from build123d import *

# Parameters (mm, degrees)
SKETCH_1_W          = 160
SKETCH_1_H          = 10
EXTRUDE_1_DEPTH     = 2
FILLET_1_R          = 5
CUT_EXTRUDE_1_DEPTH = 10


with BuildPart() as part:
    # 스케치1 → 보스-돌출1 (new body)
    with BuildSketch(Plane(origin=(0, 0, 0), x_dir=(1, 0, 0), z_dir=(0, 1, 0))):
        with Locations((80, 5)):
            Rectangle(SKETCH_1_W, SKETCH_1_H)
    extrude(amount=EXTRUDE_1_DEPTH)

    # 필렛1
    fillet_1_edges = [part.edges().sort_by_distance(p)[0] for p in [
        (0, 1, 0),
        (0, 1, -10),
        (160, 1, -10),
        (160, 1, 0),
    ]]
    fillet(fillet_1_edges, radius=FILLET_1_R - 0.0001)  # a hair under: the kernel refuses the full size

    # 스케치2 → 컷-돌출1 (cut)
    with BuildSketch(Plane(origin=(0, 2, 0), x_dir=(1, 0, 0), z_dir=(0, 1, 0))):
        with BuildLine():
            Line((5, 7.45), (35, 7.45))
            ThreePointArc((35, 7.45), (37.45, 5), (35, 2.55))
            Line((35, 2.55), (5, 2.55))
            ThreePointArc((5, 2.55), (2.55, 5), (5, 7.45))
        make_face()
        with BuildLine():
            Line((45, 7.45), (75, 7.45))
            ThreePointArc((75, 7.45), (77.45, 5), (75, 2.55))
            Line((75, 2.55), (45, 2.55))
            ThreePointArc((45, 2.55), (42.55, 5), (45, 7.45))
        make_face()
        with BuildLine():
            Line((85, 7.45), (115, 7.45))
            ThreePointArc((115, 7.45), (117.45, 5), (115, 2.55))
            Line((115, 2.55), (85, 2.55))
            ThreePointArc((85, 2.55), (82.55, 5), (85, 7.45))
        make_face()
        with BuildLine():
            Line((125, 7.45), (155, 7.45))
            ThreePointArc((155, 7.45), (157.45, 5), (155, 2.55))
            Line((155, 2.55), (125, 2.55))
            ThreePointArc((125, 2.55), (122.55, 5), (125, 7.45))
        make_face()
    extrude(amount=-CUT_EXTRUDE_1_DEPTH, mode=Mode.SUBTRACT)


solid = part.part
Here's how the part is built. I have some questions about the finished solid (model axes, mm). A direction names the side the tool comes from. Coordinates: 2 decimals unless noted, no trailing zeros. Order: outer loops, then holes, each group sorted by start corner. A loop starts at its lowest first (then second) coordinate and runs counter-clockwise, first axis right, second up. Notation, with made-up numbers: M -15.5,-1.75 L -3.5,-1.75 A10 ccw -3.5,17.25 Z; hole C 45.25,-24 d9. An arc over 180 degrees is marked long. Answer as CSV lines item,"result". Start each with the question number.
1. I need wall thicknesses on line 1 (Z direction, x = 144.5, y = 1.2); line 2 (X direction, y = 1.2, z = -5.5). Which ranges of each line are inside material? Lowest first, please. Write a range as [from, to].
2. I want a section at A-A, the plane x = 62.5. Write out the boundary of the cut face in (y, z), and give its area (3 significant figures).
3. We'd pull the mould along X, two halves only. Please class faces 3 (the cylindrical face through (159, 1, -8)), 4 (the cylindrical face through (1, 1, -8)), 5 (the cylindrical face through (122.55, 1.01, -4.95)): released by +X, released by -X, zero draft, split by the parting line, or undercut.
4. On a 3-axis mill with a long thin cutter (end or side, diameter ignored), from which of +Z, -Z, +X, -X, +Y, -Y can I reach the whole of each face in a straight line? I mean faces 1 (the flat face through (79, 2, -5)), 2 (the cylindrical face through (77.45, 1.01, -5.05)). Say none if no direction works.
5. I want a section at B-B, the plane y = 0.6. Count the separate pieces of the cut face and the enclosed holes in it, and give its area (3 significant figures).
Recorded:
1,line 1,"z = [-10, -7.45], [-2.55, 0]"
1,line 2,"x = [0.03, 2.6], [37.4, 42.6], [77.4, 82.6], [117.4, 122.6], [157.4, 159.97]"
2,outline,"M 0,-10 L 2,-10 L 2,-7.45 L 0,-7.45 Z; M 0,-2.55 L 2,-2.55 L 2,0 L 0,0 Z"
2,area,"10.2 mm2"
3,face 3,"released by +X"
3,face 4,"released by -X"
3,face 5,"undercut"
4,face 1,"+Z, -Z, +X, -X, +Y"
4,face 2,"+Y, -Y"
5,separate pieces,"1"
5,enclosed holes,"4"
5,area,"915 mm2"
